Here's how the part is built. I have some questions about the finished solid (model axes, mm). Give positions to 0.01 mm unless a question says otherwise; leave off trailing zeros. Write each loop counter-clockwise with the first axis right and the second up, starting at its lowest first coordinate (ties: lowest second). Pieces come first, ordered by that corner, then holes. Notation, with made-up numbers: (40, 60.25) -> (52, 60.25) arc R25 ccw to (52, 91.25) -> close; hole circle Ø4 at (-8, -26). An arc over 180 degrees is marked (long way). Return JSON: item names as keys, results as strings.
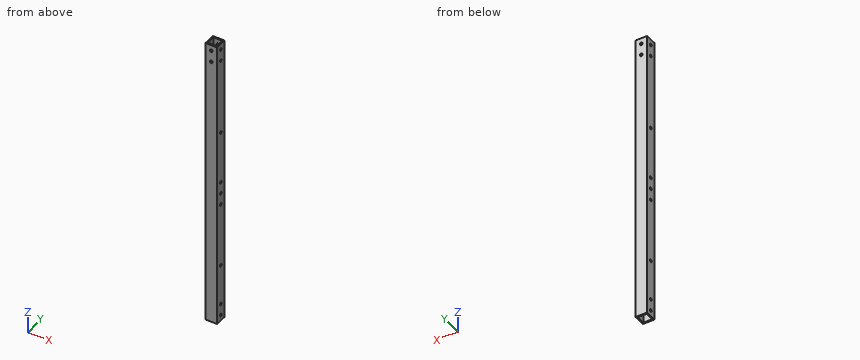
Autodesk Inventor part; units mm, degrees
ref_plane "YZ Plane" through (0, 0, 0) normal (1, 0, 0) x (0, 1, 0)
ref_plane "XZ Plane" through (0, 0, 0) normal (0, 1, 0) x (-1, 0, 0)
ref_plane "XY Plane" through (0, 0, 0) normal (0, 0, 1) x (1, 0, 0)
sketch "Sketch1" plane through (0, 0, 0) normal (0, 0, 1) x (1, 0, 0)
  line L0 (0, 0) -> (25.4, 0)
  line L1 (25.4, 0) -> (25.4, 25.4)
  line L2 (25.4, 25.4) -> (0, 25.4)
  line L3 (0, 25.4) -> (0, 0)
  line L4 (3.175, 3.175) -> (22.225, 3.175)
  line L5 (22.225, 3.175) -> (22.225, 22.225)
  line L6 (22.225, 22.225) -> (3.175, 22.225)
  line L7 (3.175, 22.225) -> (3.175, 3.175)
  dimension "d0" = 25.4
  dimension "d1" = 25.4
  dimension "d2" = 3.175
extrude "Extrusion1" add sketch "Sketch1" against normal blind 635
sketch "Sketch3" plane through (0, 25.4, 0) normal (0, 1, 0) x (1, 0, 0)
  line L0 (25.4, 0) -> (0, 0)
  point P0 (12.7, 12.7)
  point P1 (12.7, 38.1)
  dimension "d24" = 12.7
  dimension "d25" = 25.4
hole "Hole3" at (12.7, 25.4, -12.7) at (12.7, 25.4, -38.1) direction (0, -1, 0) diameter 6.35 depth 25.4 tip angle 118
sketch "Sketch4" plane through (0, 0, 0) normal (-1, 0, 0) x (0, 0, 1)
  line L0 (0, 25.4) -> (0, 0)
  point P0 (-12.7, 12.7)
  point P1 (-38.1, 12.7)
  dimension "d33" = 12.7
  dimension "d34" = 25.4
hole "Hole4" at (0, 12.7, -12.7) at (0, 12.7, -38.1) direction (1, 0, 0) diameter 6.35 depth 25.4 tip angle 118
sketch "Sketch5" plane through (25.4, 0, 0) normal (1, 0, 0) x (0, 0, -1)
  line L0 (0, 0) -> (0, 25.4)
  point P0 (317.5, 12.7)
  point P1 (342.9, 12.7)
  point P2 (368.3, 12.7)
  point P3 (596.9, 12.7)
  point P4 (622.3, 12.7)
  point P5 (647.7, 12.7)
  point P6 (812.8, 12.7)
  point P7 (508, 12.7)
  point P8 (203.2, 12.7)
  point P9 (977.9, 12.7)
  point P10 (952.5, 12.7)
  dimension "d42" = 317.5
  dimension "d43" = 25.4
  dimension "d44" = 25.4
  dimension "d45" = 25.4
  dimension "d46" = 25.4
  dimension "d47" = 228.6
  dimension "d55" = 165.1
  dimension "d56" = 139.7
  dimension "d57" = 114.3
  dimension "d58" = 25.4
  dimension "d59" = 139.7
hole "Hole5" at (25.4, 12.7, -317.5) at (25.4, 12.7, -342.9) at (25.4, 12.7, -368.3) at (25.4, 12.7, -596.9) at (25.4, 12.7, -622.3) at (25.4, 12.7, -647.7) at (25.4, 12.7, -203.2) at (25.4, 12.7, -508) at (25.4, 12.7, -812.8) at (25.4, 12.7, -952.5) at (25.4, 12.7, -977.9) direction (-1, 0, 0) diameter 6.35 depth 25.4 tip angle 118
properties part number "towermediumfrontthing"
1. For pin 1 Ø5.5 at (x, z) = (12.5, -401) entering from -Y, with a flat end and sliding along its axis, tell me the tip position at first contact or that it passes through.
Taken from the geometry:
{"pin 1": "stops at y = 0"}
2. If I drill on line 1 (Z direction, x = 12.7, y = 2.55) (3 decimals); line 2 (X direction, y = 18.25, z = -181) (3 decimals), over which ranges is the centre line in solid material (lowest first)? Write a range as [from, to].
Taken from the geometry:
{"line 1": "z = [-635, -41.275], [-34.925, -15.875], [-9.525, 0]", "line 2": "x = [0, 3.175], [22.225, 25.4]"}
3. Suppose I cut it at A-A, the plane z = -288. List the corners of the cut face in (x, y) for me (3 decimals), and give its area (3 significant figures).
Taken from the geometry:
{"outline": "(0, 0) -> (25.4, 0) -> (25.4, 25.4) -> (0, 25.4) -> close; hole (3.175, 3.175) -> (22.225, 3.175) -> (22.225, 22.225) -> (3.175, 22.225) -> close", "area": "282 mm²"}
